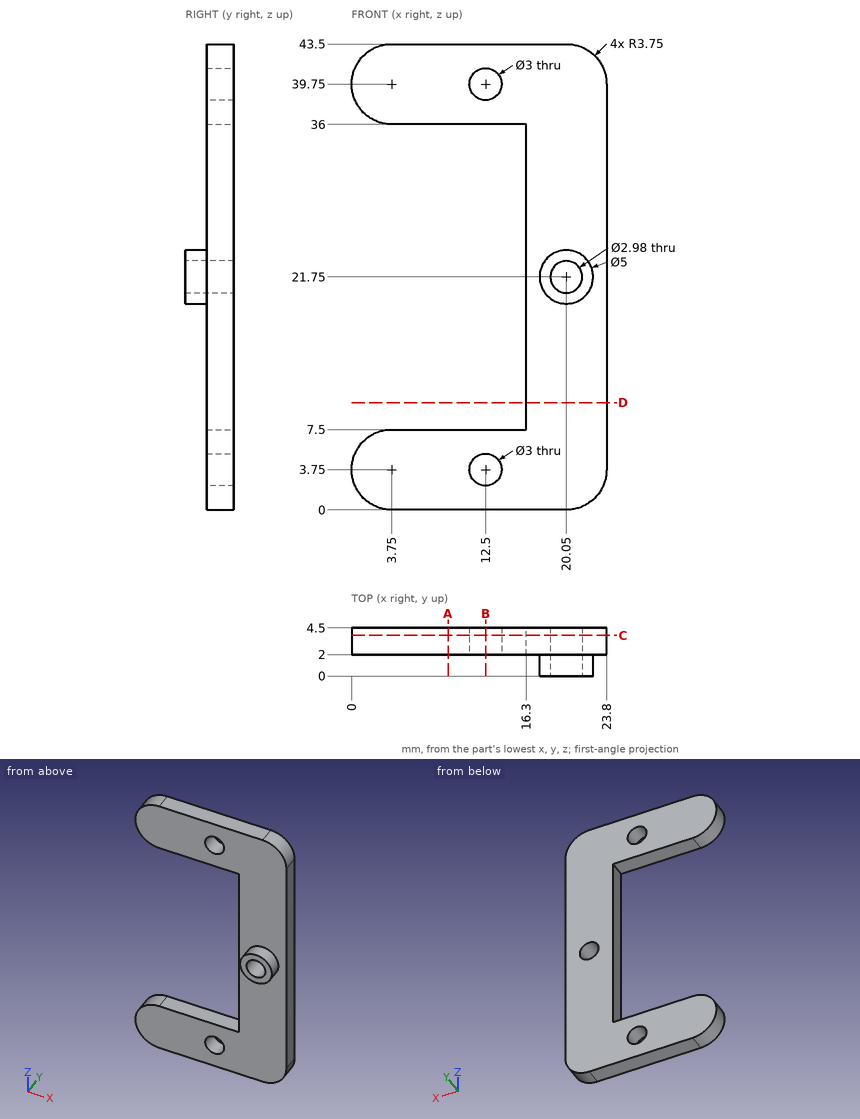
Geometry: see drawing. Coordinates: mm, zero at the bounding-box minimum. Give positions to 0.01 mm unless a question says otherwise; leave off trailing zeros. Write each loop counter-clockwise with the first axis right and the second up, starting at its lowest first coordinate (ties: lowest second). Pieces come first, ordered by that corner, then holes. Notation, with made-up numbers: M 51,77.25 L 84,77.25 A22 cw 84,116.25 Z; hole C 44.5,-18.5 d2. An arc over 180 degrees is marked long. Answer as a JSON object with one key per item and string values.
Q1. Cut plane C-C, the plane y = 3.8. Return the cut outline in (x, z).
Geometry check:
{"outline": "M 3.75,0 L 20.05,0 A3.75 ccw 23.8,3.75 L 23.8,39.75 A3.75 ccw 20.05,43.5 L 3.75,43.5 A3.75 ccw 3.75,36 L 16.3,36 L 16.3,7.5 L 3.75,7.5 A3.75 ccw Z; hole C 12.5,3.75 d3; hole C 12.5,39.75 d3; hole C 20.05,21.75 d2.98"}
Q2. Cut plane A-A, the plane x = 9. Return the cut outline in (y, z), then the cut area to 3 significant figures.
Geometry check:
{"outline": "M 2,0 L 4.5,0 L 4.5,7.5 L 2,7.5 Z; M 2,36 L 4.5,36 L 4.5,43.5 L 2,43.5 Z", "area": "37.5 mm^2"}
Q3. Ray query, line 1 along X through (y, z) = (1.3, 21.75); line 2 along X through (y, z) = (3.9, 3.75); line 3 along Z through (x, y) = (9.5, 4.1). Return the intervals inside material, ascending.
Geometry check:
{"line 1": "x = 17.55 to 18.56, 21.54 to 22.55", "line 2": "x = 0 to 11, 14 to 23.8", "line 3": "z = 0 to 7.5, 36 to 43.5"}
Q4. Cut plane B-B, the plane x = 12.5. Return the cut outline in (y, z), then the cut area to 3 significant figures.
Geometry check:
{"outline": "M 2,0 L 4.5,0 L 4.5,2.25 L 2,2.25 Z; M 2,5.25 L 4.5,5.25 L 4.5,7.5 L 2,7.5 Z; M 2,36 L 4.5,36 L 4.5,38.25 L 2,38.25 Z; M 2,41.25 L 4.5,41.25 L 4.5,43.5 L 2,43.5 Z", "area": "22.5 mm^2"}
Q5. Cut plane D-D, the plane z = 10. Return the cut outline in (x, y).
Geometry check:
{"outline": "M 16.3,2 L 23.8,2 L 23.8,4.5 L 16.3,4.5 Z"}
Q6. Contact query for flat-ended pins moving along their axis: P1, Ø5, axis at x = 12.5, z = 39.75, coming from the -Y side; P2, Ø1, axis at x = 6.5, y = 1, coming from the +Z side; P3, Ø1.2, axis at y = 4, z = 20.5, coming from the -X side. Output: stop coordinate, or through.
Geometry check:
{"P1": "stops at y = 2", "P2": "passes through", "P3": "stops at x = 16.3"}
